Check sheet for the modelled part. Datum: model origin and axes. Units: mm. Give positions to 0.01 mm unless a question says otherwise; leave off trailing zeros. Loops run counter-clockwise (first coordinate to the right, second up) from the corner with the lowest first, then second, coordinate; pieces in that order, holes last. Notation, with made-up numbers: M 29.25,59.5 L 68.25,59.5 A20 ccw 68.25,72.5 Z; hole C 63.5,86.25 d4. An arc over 180 degrees is marked long. Use one line per item in the form item = value.
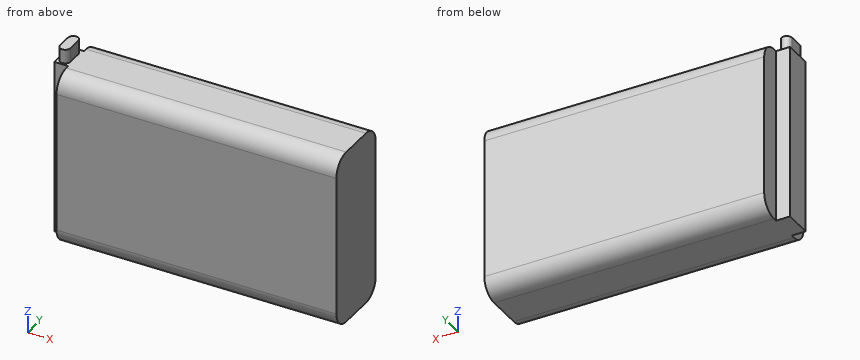
from build123d import *

# Parameters (mm, degrees)
SKETCH_1_W      = 40
SKETCH_1_H      = 25
EXTRUDE_1_DEPTH = 10
FILLET_1_R      = 2.5
SKETCH_2_W      = 25
SKETCH_2_H      = 4
EXTRUDE_2_DEPTH = 2
EXTRUDE_3_DEPTH = 2


with BuildPart() as part:
    # 草图1 → 凸台-拉伸1 (new body)
    with BuildSketch(Plane(origin=(0, 0, 0), x_dir=(1, 0, 0), z_dir=(0, 1, 0))):
        with Locations((20, 12.5)):
            Rectangle(SKETCH_1_W, SKETCH_1_H)
    extrude(amount=EXTRUDE_1_DEPTH)

    # 圆角1
    fillet_1_edges = [part.edges().sort_by_distance(p)[0] for p in [
        (20, 10, -25),
        (20, 0, -25),
        (20, 0, 0),
        (20, 10, 0),
    ]]
    fillet(fillet_1_edges, radius=FILLET_1_R)

    # 草图2 → 凸台-拉伸2 (add)
    with BuildSketch(Plane.ZY):
        with Locations((-12.5, 5)):
            Rectangle(SKETCH_2_W, SKETCH_2_H)
    extrude(amount=EXTRUDE_2_DEPTH)

    # 草图3 → 凸台-拉伸3 (add)
    with BuildSketch(Plane.XY):
        with BuildLine():
            Line((-0.26, 6), (-0.26, 4))
            ThreePointArc((-0.26, 4), (-1, 3.26), (-1.74, 4))
            Line((-1.74, 4), (-1.74, 6))
            ThreePointArc((-1.74, 6), (-1, 6.74), (-0.26, 6))
        make_face()
    extrude(amount=EXTRUDE_3_DEPTH)


solid = part.part
1) Depth check by flat-ended pin: pin 1 Ø1.6 at (y, z) = (5, 1) entering from -X; pin 2 Ø0.9 at (y, z) = (9, -7) entering from -X; pin 3 Ø0.6 at (x, z) = (-1, -11.5) entering from +Y. Enter the tip coordinate at first touch or a pass-through.
Evaluation:
pin_1 = -1.74
pin_2 = 0
pin_3 = 7
2) Section check D-D (y = 8.75). Record the cut outline in (x, z), then the cut area to 3 significant figures.
Evaluation:
outline = M 0,-24.67 L 40,-24.67 L 40,-0.33 L 0,-0.33 Z
area = 973 mm^2
3) Section check A-A (x = 5.5). Record the cut outline in (y, z), then the cut area to 3 significant figures.
Evaluation:
outline = M 0,-22.5 A2.5 ccw 2.5,-25 L 7.5,-25 A2.5 ccw 10,-22.5 L 10,-2.5 A2.5 ccw 7.5,0 L 2.5,0 A2.5 ccw 0,-2.5 Z
area = 245 mm^2
4) Section check B-B (z = -16.75). Record the cut outline in (x, y).
Evaluation:
outline = M -2,3 L 0,3 L 0,0 L 40,0 L 40,10 L 0,10 L 0,7 L -2,7 Z
5) Scan lines: line 1 (X direction, y = 9.25, z = -18.25); line 2 (Z direction, x = 9, y = 4); line 3 (Z direction, x = 23.5, y = 0.5). Record each from-to range of solid material in increasing order.
Evaluation:
line_1 = 0 to 40
line_2 = -25 to 0
line_3 = -24 to -1
6) Section check C-C (y = 1.5). Record the cut outline in (x, z).
Evaluation:
outline = M 0,-24.79 L 40,-24.79 L 40,-0.21 L 0,-0.21 Z
